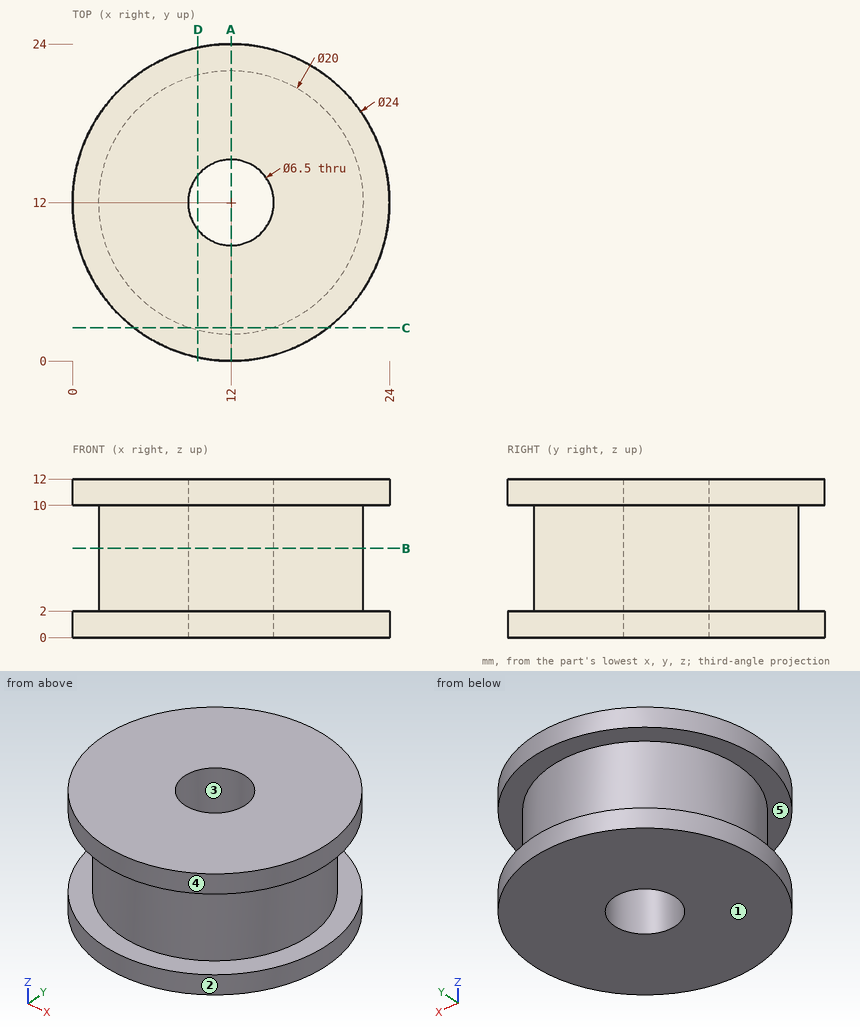
Job drawing, mm, ordinate dimensions from the low corner. One solid piece. A direction names the side the tool comes from. Round coordinates to 2 decimals unless told otherwise and drop trailing zeros. Order: outer loops, then holes, each group sorted by start corner. A loop starts at its lowest first (then second) coordinate and runs counter-clockwise, first axis right, second up. Notation, with made-up numbers: M 72,86 L 84,86 A30 cw 84,111 Z; hole C 2,-29.5 d4. An arc over 180 degrees is marked long. Write each question's results on one line, items separated by ' | '. Start each with the question number.
(1) Saw through at A-A, the plane x = 12. Give the cut face in (y, z).
(2) Saw through at C-C, the plane y = 2.5. Give the cut face in (x, z).
(3) Drop flat-ended pins along their axis: pin 1 (6 mm diameter, centred on x = 7.5, z = 2.5, fed in from +Y); pin 2 (4 mm diameter, centred on x = 13.5, z = 6.5, fed in from -Y); pin 3 (2 mm diameter, centred on y = 18, z = 5, fed in from -X). Give the stop position or say it passes through.
(4) Two-plate mould, pull along X, no slides. Class the marked faces 1, 2 and 3: pulls with the +X half, pulls with the -X half, needs draft (parallel to the pull), parting line crosses it, or undercut.
(5) Probe probe 1 along Y at (x, z) = (12, 6.5); probe 2 along Z at (x, y) = (1.75, 9.5); probe 3 along Y at (x, z) = (14.25, 11.75). List the from-to ranges inside material, lowest first. Write a range as from..to.
(6) Saw through at D-D, the plane x = 9.5. Give the cut face in (y, z), then the cut area to 3 significant figures.
(7) Saw through at B-B, the plane z = 6.75. Give the cut face in (x, y), then the cut area to 3 significant figures.
(8) Which spindle directions (+Z, -Z, +X, -X, +Y, -Y) get a long thin tool onto all of the face, cutting with end or side? Do the marked faces 4 and 5. Say none if no direction does.
Established:
1) outline: M 0,0 L 8.75,0 L 8.75,12 L 0,12 L 0,10 L 2,10 L 2,2 L 0,2 Z; M 15.25,0 L 24,0 L 24,2 L 22,2 L 22,10 L 24,10 L 24,12 L 15.25,12 Z
2) outline: M 4.67,0 L 19.33,0 L 19.33,2 L 15.12,2 L 15.12,10 L 19.33,10 L 19.33,12 L 4.67,12 L 4.67,10 L 8.88,10 L 8.88,2 L 4.67,2 Z
3) pin 1: stops at y = 23.9 | pin 2: stops at y = 2 | pin 3: stops at x = 3.34
4) face 1: needs draft | face 2: parting line crosses it | face 3: undercut
5) probe 1: y = 2..8.75, 15.25..22 | probe 2: z = 0..2, 10..12 | probe 3: y = 0.21..9.65, 14.35..23.79
6) outline: M 0.26,0 L 9.92,0 L 9.92,12 L 0.26,12 L 0.26,10 L 2.32,10 L 2.32,2 L 0.26,2 Z; M 14.08,0 L 23.74,0 L 23.74,2 L 21.68,2 L 21.68,10 L 23.74,10 L 23.74,12 L 14.08,12 Z | area: 199 mm^2
7) outline: C 12,12 d20; hole C 12,12 d6.5 | area: 281 mm^2
8) face 4: +Z, -Z | face 5: none
